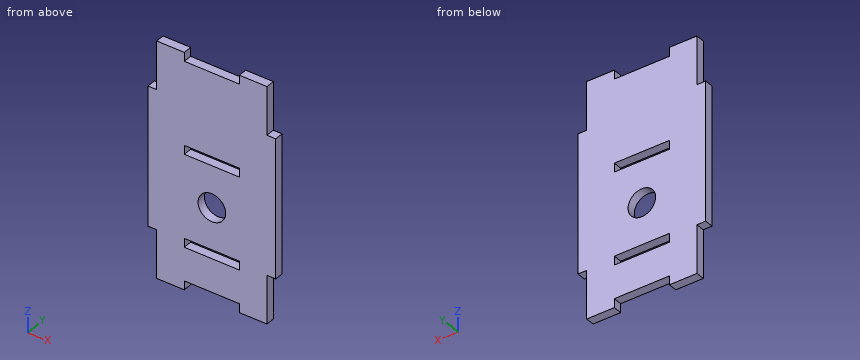
Autodesk Inventor part; units mm, degrees
ref_plane "YZ Plane" through (0, 0, 0) normal (1, 0, 0) x (0, 1, 0)
ref_plane "XZ Plane" through (0, 0, 0) normal (0, 1, 0) x (-1, 0, 0)
ref_plane "XY Plane" through (0, 0, 0) normal (0, 0, 1) x (1, 0, 0)
sketch "Boceto1" plane through (0, 0, 0) normal (0, 1, 0) x (-1, 0, 0)
  circle A0 centre (0, 0) radius 5
  line L0 (20, 51.36) -> (-20, 51.36)
  line L1 (-20, 51.36) -> (-20, -33.36)
  line L2 (-20, -33.36) -> (20, -33.36)
  line L3 (20, -33.36) -> (20, 51.36)
  line L4 (10, -15) -> (-10, -15)
  line L5 (-10, -15) -> (-10, -18.18)
  line L6 (-10, -18.18) -> (10, -18.18)
  line L7 (10, -18.18) -> (10, -15)
  line L8 (10, -15) -> (-10, -18.18) construction
  line L9 (-10, -15) -> (10, -18.18) construction
  line L10 (10, -30.18) -> (-10, -30.18)
  line L11 (-10, -30.18) -> (-10, -33.36)
  line L12 (-10, -33.36) -> (10, -33.36)
  line L13 (10, -33.36) -> (10, -30.18)
  line L14 (10, -30.18) -> (-10, -33.36) construction
  line L15 (-10, -30.18) -> (10, -33.36) construction
  line L16 (10, 18.18) -> (-10, 18.18)
  line L17 (-10, 18.18) -> (-10, 15)
  line L18 (-10, 15) -> (10, 15)
  line L19 (10, 15) -> (10, 18.18)
  line L20 (10, 18.18) -> (-10, 15) construction
  line L21 (-10, 18.18) -> (10, 15) construction
  line L22 (10, 51.36) -> (-10, 51.36)
  line L23 (-10, 51.36) -> (-10, 48.18)
  line L24 (-10, 48.18) -> (10, 48.18)
  line L25 (10, 48.18) -> (10, 51.36)
  line L26 (10, 51.36) -> (-10, 48.18) construction
  line L27 (-10, 51.36) -> (10, 48.18) construction
  line L28 (-23.18, 34) -> (-20, 34)
  line L29 (-20, 34) -> (-20, -16)
  line L30 (-20, -16) -> (-23.18, -16)
  line L31 (-23.18, -16) -> (-23.18, 34)
  line L32 (-23.18, 34) -> (-20, -16) construction
  line L33 (-20, 34) -> (-23.18, -16) construction
  line L34 (20, 34) -> (23.18, 34)
  line L35 (23.18, 34) -> (23.18, -16)
  line L36 (23.18, -16) -> (20, -16)
  line L37 (20, -16) -> (20, 34)
  line L38 (20, 34) -> (23.18, -16) construction
  line L39 (23.18, 34) -> (20, -16) construction
  point P0 (0, -16.59)
  point P1 (0, -31.77)
  point P2 (0, 16.59)
  point P3 (0, 49.77)
  point P4 (-21.59, 9)
  point P5 (21.59, 9)
  dimension "d0" = 10
  dimension "d1" = 40
  dimension "d2" = 20
  dimension "d3" = 33.36
  dimension "d5" = 0
  dimension "d6" = 3.18
  dimension "d7" = 20
  dimension "d8" = 3.18
  dimension "d9" = 20
  dimension "d10" = 0
  dimension "d11" = 12
  dimension "d12" = 3.18
  dimension "d13" = 20
  dimension "d14" = 3.18
  dimension "d15" = 20
  dimension "d16" = 0
  dimension "d17" = 0
  dimension "d18" = 30
  dimension "d19" = 30
  dimension "d20" = 3.18
  dimension "d21" = 50
  dimension "d22" = 42.36
  dimension "d23" = 3.18
  dimension "d24" = 50
  dimension "d25" = 42.36
extrude "Extrusión2" add sketch "Boceto1" along normal blind 3.18 contours L3 L2 L13 L10 L11 L1 L0 L23 L24 L25 | L34 L35 L36 L3 | L1 L30 L31 L28
properties part number "HOMBRO_FONDO"
Verification items for the finished model (mm, model axes). Round coordinates to 2 decimals unless told otherwise and drop trailing zeros. Order: outer loops, then holes, each group sorted by start corner. A loop starts at its lowest first (then second) coordinate and runs counter-clockwise, first axis right, second up. Notation, with made-up numbers: (9.25, 76) - (21.25, 76) arc R19 cw to (21.25, 98) - close; hole circle Ø3 at (-15.75, -5). An arc over 180 degrees is marked (long way). Use CSV: the item, a comma, the result in double quotes.
(1) Section check A-A on z = 0. Record the boundary of the cut face in (x, y), and give its area (3 significant figures).
Entries:
outline,"(-23.18, 0) - (-5, 0) - (-5, 3.18) - (-23.18, 3.18) - close; (5, 0) - (23.18, 0) - (23.18, 3.18) - (5, 3.18) - close"
area,"116 mm^2"
(2) Section check C-C on x = 9. Record the boundary of the cut face in (y, z).
Entries:
outline,"(0, -30.18) - (3.18, -30.18) - (3.18, -18.18) - (0, -18.18) - close; (0, -15) - (3.18, -15) - (3.18, 15) - (0, 15) - close; (0, 18.18) - (3.18, 18.18) - (3.18, 48.18) - (0, 48.18) - close"
(3) Section check B-B on x = 0. Record the boundary of the cut face in (y, z).
Entries:
outline,"(0, -30.18) - (3.18, -30.18) - (3.18, -18.18) - (0, -18.18) - close; (0, -15) - (3.18, -15) - (3.18, -5) - (0, -5) - close; (0, 5) - (3.18, 5) - (3.18, 15) - (0, 15) - close; (0, 18.18) - (3.18, 18.18) - (3.18, 48.18) - (0, 48.18) - close"
(4) Gauge pin test, flat ends, axial feed: pin 1 Ø1.6 at (y, z) = (2, 43.5) entering from -X; pin 2 Ø1 at (x, y) = (-1.5, 1.5) entering from -Z; pin 3 Ø1.6 at (x, y) = (-5, 1.5) entering from +Z. Record the tip position at first contact, or that the pin passes through.
Entries:
pin 1,"x = -20"
pin 2,"z = -30.18"
pin 3,"z = 48.18"
(5) Section check D-D on y = 1.65. State how many separate pieces and enclosed holes the cut face has, and give its area (3 significant figures).
Entries:
separate pieces,"1"
enclosed holes,"3"
area,"3,370 mm^2"
(6) Thickness scan on probe 1 along Z at (x, y) = (5.5, 1.6); probe 2 along Z at (x, y) = (0, 2.25); probe 3 along Z at (x, y) = (4, 1.75). Record the ranges inside material, lowest first. Write a range as from..to.
Entries:
probe 1,"-30.18..-18.18, -15..15, 18.18..48.18"
probe 2,"-30.18..-18.18, -15..-5, 5..15, 18.18..48.18"
probe 3,"-30.18..-18.18, -15..-3, 3..15, 18.18..48.18"
